Part model, mm, in its own coordinate system. Give positions to 0.01 mm unless a question says otherwise; leave off trailing zeros. Order: outer loops, then holes, each group sorted by start corner. A loop starts at its lowest first (then second) coordinate and runs counter-clockwise, first axis right, second up.
1. Slice it at C-C on z = -67.5. List the corners of the cut face in (x, y).
2. Drop flat-ended pins along their axis: pin 1 Ø1.5 at (y, z) = (-2.5, 104.5) entering from +X; pin 2 Ø1.5 at (x, z) = (0.5, 167.5) entering from +Y; pin 3 Ø0.9 at (x, y) = (0.5, -2) entering from -Z; pin 4 Ø0.9 at (x, y) = (-0.5, -4) entering from +Z. Give the stop position or say it passes through.
3. Slice it at B-B on x = 0.05. List the corners of the cut face in (y, z), and give its area (3 significant figures).
4. Probe line 1 (Y direction, x = -1.2, z = 166); line 2 (Z direction, x = -0.8, y = 18); line 3 (Z direction, x = -1.25, y = 15.5). List the from-to ranges inside material, lowest first.
5. Slice it at A-A on y = 11.5. List the corners of the cut face in (x, z).
Autodesk Inventor part; units mm, degrees
ref_plane "YZ Plane" through (0, 0, 0) normal (1, 0, 0) x (0, 1, 0)
ref_plane "XZ Plane" through (0, 0, 0) normal (0, 1, 0) x (-1, 0, 0)
ref_plane "XY Plane" through (0, 0, 0) normal (0, 0, 1) x (1, 0, 0)
sketch "Sketch2" plane through (0, 0, 0) normal (0, 1, 0) x (-1, 0, 0)
  line L0 (-1.5, -198.6195) -> (1.5, -198.6195)
  line L1 (1.5, -198.6195) -> (1.5, 198.6195)
  line L2 (1.5, 198.6195) -> (-1.5, 198.6195)
  line L3 (-1.5, 198.6195) -> (-1.5, -198.6195)
  line L4 (-1.5, -198.6195) -> (1.5, 198.6195) construction
  line L5 (1.5, -198.6195) -> (-1.5, 198.6195) construction
  point P0 (0, 0)
  dimension "d0" = 3
  dimension "d1" = 397.239
extrude "Extrusion1" add sketch "Sketch2" along normal blind 20
sketch "Sketch4" plane through (1.5, 0, -198.6195) normal (1, 0, 0) x (0, 0, -1)
  line L0 (0, 0) -> (-397.239, 0)
  line L1 (-397.239, 0) -> (-397.239, 20)
  line L2 (-397.239, 0) -> (-397.239, 20)
  line L3 (-397.239, 20) -> (-393.7125, 20)
  line L4 (-397.239, 20) -> (0, 20)
  line L5 (-397.239, 0) -> (-393.7125, 20)
  point P0 (-198.6195, 0)
  point P1 (-329.239, 0)
  dimension "d10" = 10
extrude "Extrusion3" cut sketch "Sketch4" against normal through all
sketch "Sketch6" plane through (1.5, 0, -198.6195) normal (1, 0, 0) x (0, 0, -1)
  line L0 (-393.7125, 20) -> (0, 20)
  line L1 (-369.839, 20) -> (-363.839, 20)
  line L2 (-363.839, 20) -> (-363.839, 8)
  line L3 (-363.839, 8) -> (-369.839, 8)
  line L4 (-369.839, 8) -> (-369.839, 20)
  line L5 (-397.239, 0) -> (0, 0) construction
  line L6 (-397.239, 0) -> (-397.239, 30) construction
  point P0 (-198.6195, 0)
  dimension "d20" = 6
  dimension "d21" = 12
  dimension "d25" = 27.4
extrude "Extrusion5" cut sketch "Sketch6" against normal blind 6
sketch "Sketch7" plane through (1.5, 0, -198.6195) normal (1, 0, 0) x (0, 0, -1)
  line L0 (0, 0) -> (-397.239, 0)
  line L1 (-357.239, 0) -> (-342.239, 0)
  line L2 (-342.239, 0) -> (-342.239, -6)
  line L3 (-342.239, -6) -> (-357.239, -6)
  line L4 (-357.239, -6) -> (-357.239, 0)
  line L5 (-197.239, 0) -> (-182.239, 0)
  line L6 (-182.239, 0) -> (-182.239, -6)
  line L7 (-182.239, -6) -> (-197.239, -6)
  line L8 (-197.239, -6) -> (-197.239, 0)
  line L9 (-37.239, 0) -> (-22.239, 0)
  line L10 (-22.239, 0) -> (-22.239, -6)
  line L11 (-22.239, -6) -> (-37.239, -6)
  line L12 (-37.239, -6) -> (-37.239, 0)
  point P0 (-198.6195, 0)
  dimension "d26" = 15
  dimension "d27" = 6
  dimension "d28" = 15
  dimension "d29" = 15
  dimension "d30" = 6
  dimension "d31" = 40
  dimension "d32" = 145
  dimension "d33" = 145
extrude "Extrusion6" add sketch "Sketch7" against normal blind 3
properties part number "wall outer plunger"
Data:
1. outline: (-1.5, 0) - (1.5, 0) - (1.5, 20) - (-1.5, 20) - close
2. pin 1: passes through
2. pin 2: stops at y = 8
2. pin 3: stops at z = -176.38
2. pin 4: stops at z = 158.62
3. outline: (-6, -176.38) - (0, -176.38) - (0, -198.62) - (20, -198.62) - (20, 165.22) - (8, 165.22) - (8, 171.22) - (20, 171.22) - (20, 195.09) - (0, 198.62) - (0, 158.62) - (-6, 158.62) - (-6, 143.62) - (0, 143.62) - (0, -1.38) - (-6, -1.38) - (-6, -16.38) - (0, -16.38) - (0, -161.38) - (-6, -161.38) - close
3. area: 8,110 mm2
4. line 1: y = 0 to 8
4. line 2: z = -198.62 to 165.22, 171.22 to 195.45
4. line 3: z = -198.62 to 165.22, 171.22 to 195.89
5. outline: (-1.5, -198.62) - (1.5, -198.62) - (1.5, 165.22) - (-1.5, 165.22) - close; (-1.5, 171.22) - (1.5, 171.22) - (1.5, 196.59) - (-1.5, 196.59) - close
